from build123d import *

# Parameters (mm, degrees)
SKETCH1_W               = 10.16
SKETCH1_H               = 9.652
BOSS_EXTRUDE1_DEPTH     = 7.112
CUT_EXTRUDE1_DEPTH      = 14.021061708
CUT_EXTRUDE1_DEPTH_BACK = 14.021061708
SKETCH2_R               = 1.5875
SKETCH7_W               = 10.16
SKETCH7_H               = 9.652
BOSS_EXTRUDE3_DEPTH     = 1.27
FILLET1_R               = 0.635
FILLET3_R               = 0.635
FILLET4_R               = 0.381
CUT_EXTRUDE3_DEPTH      = 14.485940976
CUT_EXTRUDE3_DEPTH_BACK = 14.485940976
FILLET9_R               = 0.254
CUT_EXTRUDE7_DEPTH      = 9.654656319
SKETCH14_W              = 3.81
SKETCH14_H              = 3.302
BOSS_EXTRUDE4_DEPTH     = 17.78
FILLET14_R              = 1.27
FILLET15_R              = 0.254


with BuildPart() as part:
    # Sketch1 → Boss-Extrude1 (new body)
    with BuildSketch(Plane.XY):
        Rectangle(SKETCH1_W, SKETCH1_H)
        Polygon((-4.318, -3.81), (4.318, -3.81), (4.318, -1.016), (3.302, -1.016), (3.302, 2.794), (-3.302, 2.794), (-3.302, -1.016), (-4.318, -1.016), align=None, mode=Mode.SUBTRACT)
    extrude(amount=BOSS_EXTRUDE1_DEPTH)

    # Sketch2 → Cut-Extrude1 (cut, two sides: drawn at the far end of the back side and taken through both)
    with BuildSketch(Plane(origin=(0, 4.826, 0), x_dir=(1, 0, 0), z_dir=(0, 1, 0)).offset(-CUT_EXTRUDE1_DEPTH_BACK)):
        with Locations(Location((0, -2.794, 0), (0, 0, 90))):
            Circle(SKETCH2_R)
    extrude(amount=CUT_EXTRUDE1_DEPTH + CUT_EXTRUDE1_DEPTH_BACK, mode=Mode.SUBTRACT)

    # Sketch7 → Boss-Extrude3 (add)
    with BuildSketch(Plane.XY.offset(7.112)):
        Rectangle(SKETCH7_W, SKETCH7_H)
    extrude(amount=BOSS_EXTRUDE3_DEPTH)

    # Fillet1
    fillet1_edges = [part.edges().sort_by_distance(p)[0] for p in [
        (-5.08, 0, 0),
        (0, 4.826, 0),
        (5.08, 0, 0),
    ]]
    fillet(fillet1_edges, radius=FILLET1_R)

    # Fillet3
    # the kernel refuses this fillet: 0.635 mm, written as the material it takes off along each edge
    with BuildSketch(Plane(origin=(4.445, 4.191, 0.635), x_dir=(1, 0, 0), z_dir=(0, 1, 0))) as fillet3_piece_1_section:
        Polygon((0, 0), (FILLET3_R, 0), (FILLET3_R, FILLET3_R), (0, FILLET3_R), align=None)
    fillet3_piece_1 = extrude(amount=FILLET3_R, mode=Mode.PRIVATE)
    fillet3_piece_1 = fillet3_piece_1 - Plane(origin=(4.445, 4.191, 0.635), x_dir=(-0.7071067811865475, 0, 0.7071067811865475), z_dir=(0, 1, 0)) * Sphere(FILLET3_R, mode=Mode.PRIVATE)
    add(fillet3_piece_1, mode=Mode.SUBTRACT)
    with BuildSketch(Plane(origin=(-4.445, 4.191, 0.635), x_dir=(-1, 0, 0), z_dir=(0, 1, 0))) as fillet3_piece_2_section:
        Polygon((0, 0), (FILLET3_R, 0), (FILLET3_R, -FILLET3_R), (0, -FILLET3_R), align=None)
    fillet3_piece_2 = extrude(amount=FILLET3_R, mode=Mode.PRIVATE)
    fillet3_piece_2 = fillet3_piece_2 - Plane(origin=(-4.445, 4.191, 0.635), x_dir=(0.7071067811865475, 0, 0.7071067811865475), z_dir=(0, 1, 0)) * Sphere(FILLET3_R, mode=Mode.PRIVATE)
    add(fillet3_piece_2, mode=Mode.SUBTRACT)
    with BuildSketch(Plane(origin=(-4.445, -4.191, 7.747), x_dir=(0, 0, 1), z_dir=(-1, 0, 0))) as fillet3_piece_3_section:
        Polygon((0, 0), (FILLET3_R, 0), (FILLET3_R, -FILLET3_R), (0, -FILLET3_R), align=None)
    fillet3_piece_3 = extrude(amount=FILLET3_R, mode=Mode.PRIVATE)
    fillet3_piece_3 = fillet3_piece_3 - Plane(origin=(-4.445, -4.191, 7.747), x_dir=(0, 0.7071067811865475, -0.7071067811865475), z_dir=(-1, 0, 0)) * Sphere(FILLET3_R, mode=Mode.PRIVATE)
    add(fillet3_piece_3, mode=Mode.SUBTRACT)
    with BuildSketch(Plane(origin=(-4.445, 4.191, 7.747), x_dir=(-1, 0, 0), z_dir=(0, 1, 0))) as fillet3_piece_4_section:
        Polygon((0, 0), (FILLET3_R, 0), (FILLET3_R, FILLET3_R), (0, FILLET3_R), align=None)
    fillet3_piece_4 = extrude(amount=FILLET3_R, mode=Mode.PRIVATE)
    fillet3_piece_4 = fillet3_piece_4 - Plane(origin=(-4.445, 4.191, 7.747), x_dir=(0.7071067811865475, 0, -0.7071067811865475), z_dir=(0, 1, 0)) * Sphere(FILLET3_R, mode=Mode.PRIVATE)
    add(fillet3_piece_4, mode=Mode.SUBTRACT)
    with BuildSketch(Plane(origin=(4.445, -4.191, 7.747), x_dir=(1, 0, 0), z_dir=(0, 0, 1))) as fillet3_piece_5_section:
        Polygon((0, 0), (FILLET3_R, 0), (FILLET3_R, -FILLET3_R), (0, -FILLET3_R), align=None)
    fillet3_piece_5 = extrude(amount=FILLET3_R, mode=Mode.PRIVATE)
    fillet3_piece_5 = fillet3_piece_5 - Plane(origin=(4.445, -4.191, 7.747), x_dir=(-0.7071067811865476, 0.7071067811865475, 0), z_dir=(0, 0, 1)) * Sphere(FILLET3_R, mode=Mode.PRIVATE)
    add(fillet3_piece_5, mode=Mode.SUBTRACT)
    with BuildSketch(Plane(origin=(4.445, 4.191, 7.747), x_dir=(0, 0, 1), z_dir=(0, 1, 0))) as fillet3_piece_6_section:
        Polygon((0, 0), (FILLET3_R, 0), (FILLET3_R, FILLET3_R), (0, FILLET3_R), align=None)
    fillet3_piece_6 = extrude(amount=FILLET3_R, mode=Mode.PRIVATE)
    fillet3_piece_6 = fillet3_piece_6 - Plane(origin=(4.445, 4.191, 7.747), x_dir=(-0.7071067811865475, 0, -0.7071067811865475), z_dir=(0, 1, 0)) * Sphere(FILLET3_R, mode=Mode.PRIVATE)
    add(fillet3_piece_6, mode=Mode.SUBTRACT)
    with BuildSketch(Plane(origin=(-5.08, -4.191, 8.382), x_dir=(0, 0, -1), z_dir=(0, 1, 0))) as fillet3_piece_7:
        with BuildLine():
            CenterArc((FILLET3_R, -FILLET3_R), FILLET3_R, 90, 90)
            Line((0, -FILLET3_R), (0, 0))
            Line((0, 0), (FILLET3_R, 0))
        make_face()
    extrude(amount=8.382, mode=Mode.SUBTRACT)
    with BuildSketch(Plane(origin=(4.445, -4.826, 8.382), x_dir=(0, 1, 0), z_dir=(-1, 0, 0)), Plane(origin=(4.445, -4.826, 0), x_dir=(0, 0, 1), z_dir=(-1, 0, 0))) as fillet3_piece_8:
        with BuildLine():
            CenterArc((FILLET3_R, FILLET3_R), FILLET3_R, 180, 90)
            Line((0, FILLET3_R), (0, 0))
            Line((0, 0), (FILLET3_R, 0))
        make_face()
    extrude(amount=8.89, mode=Mode.SUBTRACT)
    with BuildSketch(Plane(origin=(5.08, 4.191, 8.382), x_dir=(-1, 0, 0), z_dir=(0, -1, 0))) as fillet3_piece_9:
        with BuildLine():
            CenterArc((FILLET3_R, FILLET3_R), FILLET3_R, 180, 90)
            Line((0, FILLET3_R), (0, 0))
            Line((0, 0), (FILLET3_R, 0))
        make_face()
    extrude(amount=8.382, mode=Mode.SUBTRACT)
    with BuildSketch(Plane(origin=(-4.445, 4.826, 8.382), x_dir=(0, 0, -1), z_dir=(1, 0, 0))) as fillet3_piece_10:
        with BuildLine():
            CenterArc((FILLET3_R, -FILLET3_R), FILLET3_R, 90, 90)
            Line((0, -FILLET3_R), (0, 0))
            Line((0, 0), (FILLET3_R, 0))
        make_face()
    extrude(amount=8.89, mode=Mode.SUBTRACT)
    with BuildSketch(Plane(origin=(4.445, -4.826, 0.635), x_dir=(0, 0, -1), z_dir=(-1, 0, 0))) as fillet3_piece_11:
        with BuildLine():
            CenterArc((0.635 - FILLET3_R, -FILLET3_R), FILLET3_R, 0, 90)
            Line((0.635, -FILLET3_R), (0.635, 0))
            Line((0.635, 0), (0.635 - FILLET3_R, 0))
        make_face()
    revolve(axis=Axis((4.445, -4.826, 0.635), (0, -1, 0)), revolution_arc=90, mode=Mode.SUBTRACT)
    with BuildSketch(Plane(origin=(-4.445, -4.826, 0.635), x_dir=(0, 0, -1), z_dir=(1, 0, 0))) as fillet3_piece_12:
        with BuildLine():
            CenterArc((0.635 - FILLET3_R, FILLET3_R), FILLET3_R, 270, 90)
            Line((0.635, FILLET3_R), (0.635, 0))
            Line((0.635, 0), (0.635 - FILLET3_R, 0))
        make_face()
    revolve(axis=Axis((-4.445, -4.826, 0.635), (0, 1, 0)), revolution_arc=90, mode=Mode.SUBTRACT)
    with BuildSketch(Plane(origin=(5.08, -4.826, 7.747), x_dir=(0, 1, 0), z_dir=(0, 0, -1)), Plane(origin=(-5.08, -4.826, 0.635), x_dir=(0, 1, 0), z_dir=(0, 0, 1)), Plane(origin=(-5.08, 4.826, 0.635), x_dir=(1, 0, 0), z_dir=(0, 0, 1)), Plane(origin=(5.08, 4.826, 7.747), x_dir=(-1, 0, 0), z_dir=(0, 0, -1))) as fillet3_piece_13:
        with BuildLine():
            CenterArc((FILLET3_R, -FILLET3_R), FILLET3_R, 90, 90)
            Line((0, -FILLET3_R), (0, 0))
            Line((0, 0), (FILLET3_R, 0))
        make_face()
    extrude(amount=7.112, mode=Mode.SUBTRACT)

    # Fillet4
    fillet4_edges = [part.edges().sort_by_distance(p)[0] for p in [
        (3.302, -1.016, 3.556),
        (-3.302, -1.016, 3.556),
    ]]
    fillet(fillet4_edges, radius=FILLET4_R)

    # Sketch11 → Cut-Extrude3 (cut, two sides: drawn at the far end of the back side and taken through both)
    with BuildSketch(Plane.ZY.offset(-4.318).offset(-CUT_EXTRUDE3_DEPTH_BACK)):
        Polygon((0, -3.81), (5.08, -3.81), (5.08, -4.064), (10.16, -4.826), (0, -4.826), align=None)
    extrude(amount=CUT_EXTRUDE3_DEPTH + CUT_EXTRUDE3_DEPTH_BACK, mode=Mode.SUBTRACT)

    # Fillet9
    fillet9_edges = [part.edges().sort_by_distance(p)[0] for p in [
        (-4.318, -3.81, 6.096),
        (4.318, -3.81, 6.096),
        (0, -3.81, 7.112),
    ]]
    fillet(fillet9_edges, radius=FILLET9_R)

    # Sketch13 → Cut-Extrude7 (cut, through all)
    with BuildSketch(Plane(origin=(0, 0, 5.08), x_dir=(-1, 0, 0), z_dir=(0, 0, -1))):
        Polygon((-5.08, -3.81), (-5.08, -4.826), (-2.032, -4.826), align=None)
        Polygon((5.08, -3.81), (5.08, -4.826), (2.032, -4.826), align=None)
    extrude(amount=-CUT_EXTRUDE7_DEPTH, mode=Mode.SUBTRACT)

    # Sketch14 → Boss-Extrude4 (add)
    with BuildSketch(Plane.XY.offset(8.382)):
        Rectangle(SKETCH14_W, SKETCH14_H)
    extrude(amount=BOSS_EXTRUDE4_DEPTH)

    # Fillet14
    fillet14_edges = [part.edges().sort_by_distance(p)[0] for p in [
        (0, 1.651, 8.382),
        (-1.905, 0, 8.382),
        (0, -1.651, 8.382),
        (1.905, 0, 8.382),
    ]]
    fillet(fillet14_edges, radius=FILLET14_R)

    # Fillet15
    fillet15_edges = [part.edges().sort_by_distance(p)[0] for p in [
        (1.905, 1.651, 17.907),
        (-1.905, 1.651, 17.907),
        (-1.905, -1.651, 17.907),
        (1.905, -1.651, 17.907),
        (0, 1.651, 26.162),
        (-1.905, 0, 26.162),
        (0, -1.651, 26.162),
        (1.905, 0, 26.162),
        (2.354517888, 2.100517888, 8.682614059),
        (2.354517888, -2.100517888, 8.682614059),
        (-2.354517888, 2.100517888, 8.682614059),
        (-2.354517888, -2.100517888, 8.682614059),
    ]]
    fillet(fillet15_edges, radius=FILLET15_R)


solid = part.part
Geometry check sheet. Reference: the model listing, model coordinates, mm. A direction names the side the tool comes from. Round coordinates to 2 decimals unless told otherwise and drop trailing zeros. Order: outer loops, then holes, each group sorted by start corner. A loop starts at its lowest first (then second) coordinate and runs counter-clockwise, first axis right, second up. Notation, with made-up numbers: M -9,68 L 1,68 A20 ccw 1,74 Z; hole C 87,52 d8. An arc over 180 degrees is marked long. Answer in a Markdown table with one row per item.
(1) Sectioned sample at C-C, the plane y = 0. Record the cut outline in (x, z) (3 decimals).
Responses:
| item | result |
|---|---|
| outline | M -5.08,0.635 A0.635 ccw -4.445,0 L -3.302,0 L -3.302,7.112 L 3.302,7.112 L 3.302,0 L 4.445,0 A0.635 ccw 5.08,0.635 L 5.08,7.747 A0.635 ccw 4.445,8.382 L 3.175,8.382 A1.27 cw 1.905,9.652 L 1.905,25.908 A0.254 ccw 1.651,26.162 L -1.651,26.162 A0.254 ccw -1.905,25.908 L -1.905,9.652 A1.27 cw -3.175,8.382 L -4.445,8.382 A0.635 ccw -5.08,7.747 Z |
(2) Scan lines: probe 1 along X at (y, z) = (4, 2.75); probe 2 along X at (y, z) = (1.5, 6.5); probe 3 along X at (y, z) = (1, 15) (3 decimals). Record each from-to range of solid material in increasing order. Write a range as from..to.
Responses:
| item | result |
|---|---|
| probe 1 | x = -5.08..-1.59, 1.59..5.08 |
| probe 2 | x = -5.08..-3.3, 3.3..5.08 |
| probe 3 | x = -1.905..1.905 |
(3) Sectioned sample at B-B, the plane z = 24.5. Record the cut outline in (x, y) (3 decimals).
Responses:
| item | result |
|---|---|
| outline | M -1.905,-1.397 A0.254 ccw -1.651,-1.651 L 1.651,-1.651 A0.254 ccw 1.905,-1.397 L 1.905,1.397 A0.254 ccw 1.651,1.651 L -1.651,1.651 A0.254 ccw -1.905,1.397 Z |
(4) Draft check along X on faces 4 (the face through (4.318, -2, 4)), 5 (the face through (4.21, -4.1, 7.07)), 6 (the face through (0, 1.651, 18)). Enter one of: released by +X, released by -X, zero draft, split by the parting line, or undercut.
Responses:
| item | result |
|---|---|
| face 4 | undercut |
| face 5 | released by +X |
| face 6 | zero draft |
(5) Sectioned sample at D-D, the plane x = 1.25. Record the cut outline in (y, z) (3 decimals).
Responses:
| item | result |
|---|---|
| outline | M -4.543,8.275 L -4.064,5.08 L -3.81,5.08 L -3.81,6.858 A0.254 cw -3.556,7.112 L 2.794,7.112 L 2.794,3.773 L 4.826,3.773 L 4.826,7.747 A0.635 ccw 4.191,8.382 L 2.921,8.382 A1.27 cw 1.651,9.652 L 1.651,25.908 A0.254 ccw 1.397,26.162 L -1.397,26.162 A0.254 ccw -1.651,25.908 L -1.651,9.652 A1.27 cw -2.921,8.382 L -4.191,8.382 A0.635 ccw Z; M 2.794,0 L 4.191,0 A0.635 ccw 4.826,0.635 L 4.826,1.815 L 2.794,1.815 Z |
(6) Tool access check on faces 1 (the face through (0, 2.794, 5)), 2 (the face through (1.905, 0, 18)), 3 (the face through (-1.905, 0, 18)). Record the directions out of +Z, -Z, +X, -X, +Y, -Y that give a thin tool (end or side, any length) a straight path to the whole face; none if there is none.
Responses:
| item | result |
|---|---|
| face 1 | -Z |
| face 2 | +Z, +X, +Y, -Y |
| face 3 | +Z, -X, +Y, -Y |
(7) Go/stop test with flat-tipped pins: P1, Ø5, axis at x = -1, z = 15.5, coming from the +Y side; P2, Ø0.6, axis at x = -1.5, y = -4, coming from the -Z side; P3, Ø0.8, axis at x = 5, z = 3.5, coming from the -Y side. Record where each tip stops, or that it passes through.
Responses:
| item | result |
|---|---|
| P1 | stops at y = 1.65 |
| P2 | stops at z = 5.08 |
| P3 | stops at y = -3.81 |
